Geometry check sheet. Reference: the model listing, model coordinates, mm. A direction names the side the tool comes from. Coordinates: 2 decimals unless noted, no trailing zeros. Loops run counter-clockwise (first coordinate to the right, second up) from the corner with the lowest first, then second, coordinate; pieces in that order, holes last. Notation, with made-up numbers: (19.25, 37.5) -> (48.25, 37.5) arc R18 cw to (48.25, 69.5) -> close; hole circle Ø5 at (-4, 68). An arc over 180 degrees is marked (long way). Answer as a JSON object with one key per item and string values.
from build123d import *

# Parameters (mm, degrees)
CUT_EXTRUDE1_START = 2
SKETCH2_W          = 10
SKETCH2_H          = 3
CUT_EXTRUDE1_DEPTH = 1.4


with BuildPart() as part:
    # Sketch1 → Revolve1 (revolve)
    with BuildSketch(Plane.XY, mode=Mode.PRIVATE) as revolve1_sk:
        Polygon((0, 0), (0, 3), (6.5, 3), (16.94, 3), (16.94, 5), (21.87, 5), (31.55, 5), (32.55, 6), (44.55, 6), (44.55, 6.5), (50.75, 6.5), (50.75, 7), (56.95, 7), (56.95, 7.5), (63.15, 7.5), (63.15, 8), (69.35, 8), (69.35, 8.5), (91.75, 8.5), (94.25, 6), (120.06, 6), (132.06, 6), (132.06, 4), (138.56, 4), (138.56, 0), align=None)
    revolve(revolve1_sk.sketch.rotate(Axis((0, 0, 0), (1, 0, 0)), 90), axis=Axis((0, 0, 0), (1, 0, 0)))

    # Sketch2 → Cut-Extrude1 (cut)
    with BuildSketch(Plane.XY.offset(3).offset(CUT_EXTRUDE1_START)):
        with Locations((26.55, 0)):
            Rectangle(SKETCH2_W, SKETCH2_H)
    extrude(amount=-CUT_EXTRUDE1_DEPTH, mode=Mode.SUBTRACT)


solid = part.part
1. Thickness scan on probe 1 along Y at (x, z) = (67.5, -0.5); probe 2 along X at (y, z) = (-2.5, 3.25); probe 3 along Z at (x, y) = (60, -3.75). Record the ranges inside material, lowest first. Write a range as from..to.
Evaluation:
{"probe 1": "y = -7.98..7.98", "probe 2": "x = 16.94..132.06", "probe 3": "z = -6.5..6.5"}
2. Mould release check, pull along X, two halves, no side actions. Record for faces 4 (the face through (26, 0, 3.6)), 5 (the face through (63.15, 6, -5)), 6 (the face through (38.634, -1.802, 5.723)), 7 (the face through (132.06, 3.92, -1.42)): released by +X, released by -X, zero draft, split by the parting line, or undercut.
Evaluation:
{"face 4": "undercut", "face 5": "released by -X", "face 6": "zero draft", "face 7": "released by +X"}
3. Section check C-C, the plane x = 97.5. Record the boundary of the cut face in (y, z), then the cut area to 3 significant figures.
Evaluation:
{"outline": "circle Ø12 at (0, 0)", "area": "113 mm^2"}
4. Section check B-B, the plane x = 72. Record the boundary of the cut face in (y, z), then the cut area to 3 significant figures.
Evaluation:
{"outline": "circle Ø17 at (0, 0)", "area": "227 mm^2"}
5. Section check A-A, the plane x = 24. Record the boundary of the cut face in (y, z), then the cut area to 3 significant figures.
Evaluation:
{"outline": "(-1.5, 3.6) -> (-1.5, 4.77) arc R5 ccw (long way) to (1.5, 4.77) -> (1.5, 3.6) -> close", "area": "74.6 mm^2"}
6. Depth check by flat-ended pin: P1, Ø3, axis at x = 57.5, y = -4, coming from the +Z side; P2, Ø0.6, axis at x = 28.5, z = 4, coming from the +Y side; P3, Ø2, axis at x = 98.5, z = -3, coming from the +Y side. Enter the tip coordinate at first touch or a pass-through.
Evaluation:
{"P1": "stops at z = 7.07", "P2": "stops at y = 3.36", "P3": "stops at y = 5.66"}
7. Tool access check on faces 1 (the face through (44.55, 6, -2)), 2 (the face through (135.356, 3.905, -0.867)), 3 (the face through (0, 0, 0)). Record the directions out of +Z, -Z, +X, -X, +Y, -Y that give a thin tool (end or side, any length) a straight path to the whole face; none if there is none.
Evaluation:
{"face 1": "-X", "face 2": "+X", "face 3": "+Z, -Z, -X, +Y, -Y"}
